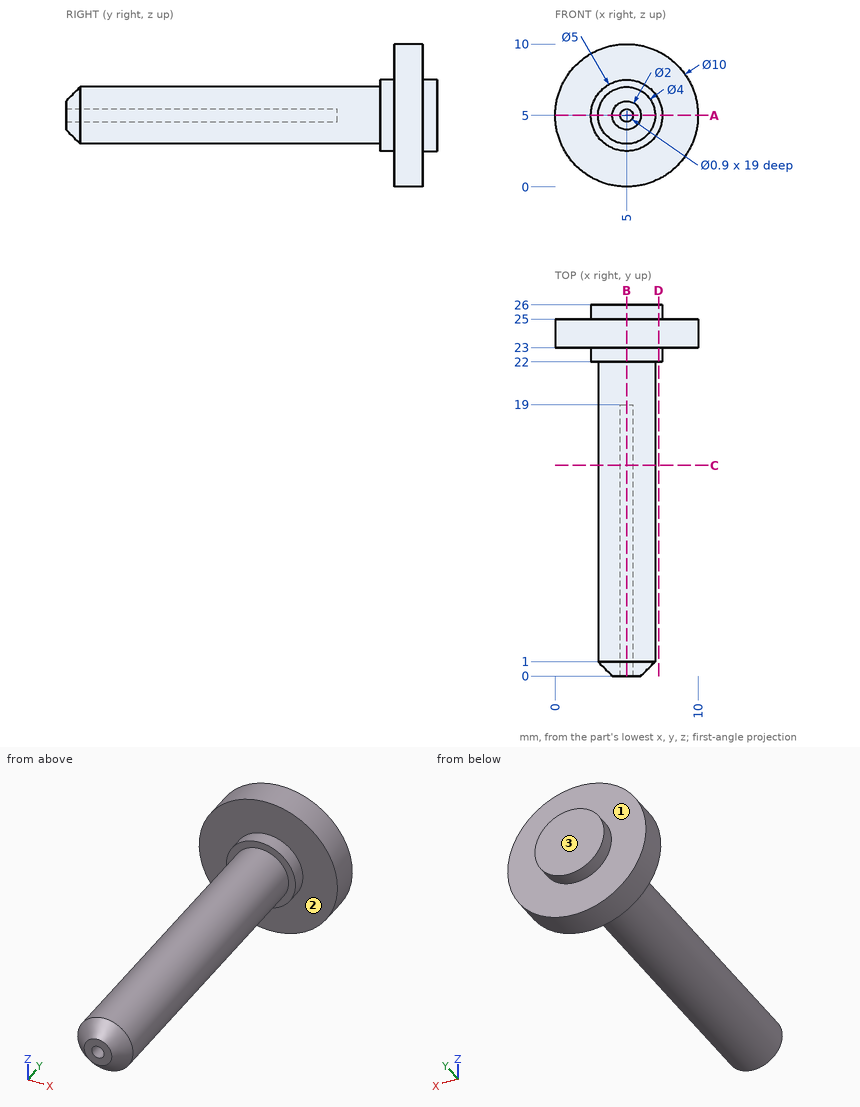
Answer from the drawing. Dimensions are ordinates in mm from the lowest x, y and z of the part. A direction names the side the tool comes from. Coordinates: 2 decimals unless noted, no trailing zeros. Loops run counter-clockwise (first coordinate to the right, second up) from the corner with the lowest first, then second, coordinate; pieces in that order, holes last.
Q1. Each of these flat-tipped pins is pushed along its axis until it touches: pin 1 Ø1.5 at (x, z) = (6.5, 2) entering from -Y; pin 2 Ø1.5 at (x, z) = (1.5, 6) entering from +Y; pin 3 Ø5 at (y, z) = (17, 7) entering from +X. Where does it stop, or does it pass through?
Q2. Which of the six approach directions +Z, -Z, +X, -X, +Y, -Y give full straight-line access (tool end or side, diameter ignored) to the marked faces 1, 2 and 3?
Q3. The part is cut by section B-B on x = 5. Write down the section's boundary in (y, z).
Q4. The part is cut by section A-A on z = 5. Write down the section's boundary in (x, y), and give its area (3 significant figures).
Q5. The part is cut by section D-D on x = 7.25. Write down the section's boundary in (y, z), and give its area (3 significant figures).
Q6. The part is cut by section C-C on y = 14.75. Write down the section's boundary in (x, z).
Q7. Consider probe 1 along Z at (x, y) = (5, 12); probe 2 along Y at (x, z) = (3.5, 8.25). Determine where each line is inside the solid, lowest interval first.
Results below:
1. pin 1: stops at y = 23
1. pin 2: stops at y = 25
1. pin 3: stops at x = 7
2. face 1: +Y
2. face 2: -Y
2. face 3: +Z, -Z, +X, -X, +Y
3. outline: (0, 4) - (1, 3) - (22, 3) - (22, 2.5) - (23, 2.5) - (23, 0) - (25, 0) - (25, 2.5) - (26, 2.5) - (26, 7.5) - (25, 7.5) - (25, 10) - (23, 10) - (23, 7.5) - (22, 7.5) - (22, 7) - (1, 7) - (0, 6) - (0, 5.45) - (19, 5.45) - (19, 4.55) - (0, 4.55) - close
4. outline: (0, 23) - (2.5, 23) - (2.5, 22) - (3, 22) - (3, 1) - (4, 0) - (4.55, 0) - (4.55, 19) - (5.45, 19) - (5.45, 0) - (6, 0) - (7, 1) - (7, 22) - (7.5, 22) - (7.5, 23) - (10, 23) - (10, 25) - (7.5, 25) - (7.5, 26) - (2.5, 26) - (2.5, 25) - (0, 25) - close
4. area: 99.9 mm2
5. outline: (22, 3.91) - (23, 3.91) - (23, 0.53) - (25, 0.53) - (25, 3.91) - (26, 3.91) - (26, 6.09) - (25, 6.09) - (25, 9.47) - (23, 9.47) - (23, 6.09) - (22, 6.09) - close
5. area: 22.2 mm2
6. outline: circle Ø4 at (5, 5); hole circle Ø0.9 at (5, 5)
7. probe 1: z = 3 to 4.55, 5.45 to 7
7. probe 2: y = 23 to 25
